The model under review builds one solid part; all positions refer to its coordinate system, in mm. Round coordinates to 2 decimals unless told otherwise and drop trailing zeros. Order: outer loops, then holes, each group sorted by start corner. A loop starts at its lowest first (then second) coordinate and runs counter-clockwise, first axis right, second up. Notation, with made-up numbers: M -13,23 L 15,23 A14 ccw 15,48 Z; hole C 54.5,0 d11. An arc over 180 degrees is marked long. One line per item, written item: value. Start each with the question number.
from build123d import *

# Parameters (mm, degrees)
SKETCH_1_R          = 2
SKETCH_1_R_2        = 1.5
EXTRUDE_1_DEPTH     = 3
SKETCH_2_W          = 80
SKETCH_2_H          = 23
SKETCH_2_H_2        = 10
CUT_EXTRUDE_1_DEPTH = 124.020323524
FILLET_1_R          = 2
FILLET_2_R          = 3
FILLET_3_R          = 1


with BuildPart() as part:
    # 草图1 → 凸台-拉伸1 (new body)
    with BuildSketch(Plane(origin=(0, 0, 0), x_dir=(1, 0, 0), z_dir=(0, 1, 0))):
        Polygon((55, 110), (55, 0), (-55, 0), (-55, 110), (-40, 110), (-40, 55), (40, 55), (40, 110), align=None)
        with Locations(Location((47.5, 32.5, 0), (0, 0, 270))):
            Circle(SKETCH_1_R, mode=Mode.SUBTRACT)
        with Locations(Location((47.5, 7.5, 0), (0, 0, 270))):
            Circle(SKETCH_1_R, mode=Mode.SUBTRACT)
        with Locations(Location((47.5, 79.5, 0), (0, 0, 270))):
            Circle(SKETCH_1_R, mode=Mode.SUBTRACT)
        with Locations(Location((47.5, 102.5, 0), (0, 0, 270))):
            Circle(SKETCH_1_R, mode=Mode.SUBTRACT)
        with Locations(Location((-47.5, 102.5, 0), (0, 0, 90))):
            Circle(SKETCH_1_R, mode=Mode.SUBTRACT)
        with Locations(Location((-47.5, 79.5, 0), (0, 0, 90))):
            Circle(SKETCH_1_R, mode=Mode.SUBTRACT)
        with Locations(Location((-47.5, 7.5, 0), (0, 0, 90))):
            Circle(SKETCH_1_R, mode=Mode.SUBTRACT)
        with Locations(Location((-47.5, 32.5, 0), (0, 0, 90))):
            Circle(SKETCH_1_R, mode=Mode.SUBTRACT)
        with Locations(Location((-32, 36, 0), (0, 0, 270))):
            Circle(SKETCH_1_R_2, mode=Mode.SUBTRACT)
        with Locations(Location((32, 36, 0), (0, 0, 90))):
            Circle(SKETCH_1_R_2, mode=Mode.SUBTRACT)
    extrude(amount=EXTRUDE_1_DEPTH)

    # 草图2 → 切除-拉伸1 (cut, through all)
    with BuildSketch(Plane(origin=(0, 3, 0), x_dir=(1, 0, 0), z_dir=(0, 1, 0))):
        with Locations((0, 21.5)):
            Rectangle(SKETCH_2_W, SKETCH_2_H)
        with Locations((0, 44)):
            Rectangle(SKETCH_2_W, SKETCH_2_H_2)
        with BuildLine():
            Line((-45.5, 70), (-45.5, 42))
            ThreePointArc((-45.5, 42), (-47.5, 40), (-49.5, 42))
            Line((-49.5, 42), (-49.5, 70))
            ThreePointArc((-49.5, 70), (-47.5, 72), (-45.5, 70))
        make_face()
        with BuildLine():
            Line((45.5, 70), (45.5, 42))
            ThreePointArc((45.5, 42), (47.5, 40), (49.5, 42))
            Line((49.5, 42), (49.5, 70))
            ThreePointArc((49.5, 70), (47.5, 72), (45.5, 70))
        make_face()
    extrude(amount=-CUT_EXTRUDE_1_DEPTH, mode=Mode.SUBTRACT)

    # 圆角1
    fillet_1_edges = [part.edges().sort_by_distance(p)[0] for p in [
        (55, 1.5, -110),
        (55, 1.5, 0),
        (-55, 1.5, 0),
        (-55, 1.5, -110),
        (-40, 1.5, -110),
        (-40, 1.5, -55),
        (40, 1.5, -55),
        (40, 1.5, -110),
    ]]
    fillet(fillet_1_edges, radius=FILLET_1_R)

    # 圆角2
    fillet_2_edges = [part.edges().sort_by_distance(p)[0] for p in [
        (-40, 1.5, -33),
        (40, 1.5, -33),
        (40, 1.5, -39),
        (-40, 1.5, -39),
    ]]
    fillet(fillet_2_edges, radius=FILLET_2_R)

    # 圆角3
    fillet_3_edges = [part.edges().sort_by_distance(p)[0] for p in [
        (-40, 1.5, -10),
        (40, 1.5, -10),
        (-40, 1.5, -49),
        (40, 1.5, -49),
    ]]
    fillet(fillet_3_edges, radius=FILLET_3_R)


solid = part.part
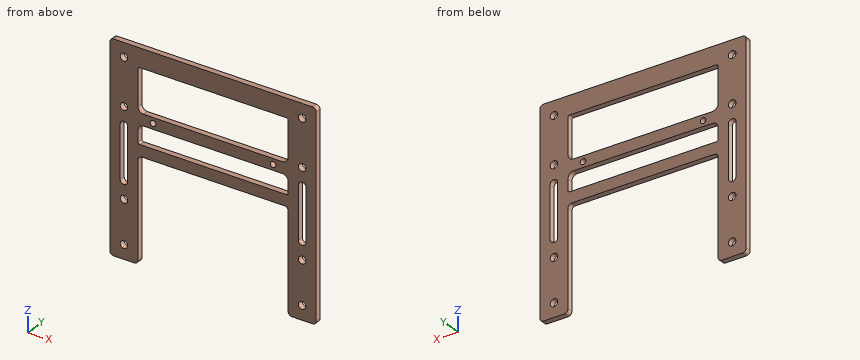
Item 1: Clearance check with a flat-ended pin moving along its axis: P1, Ø1.5, axis at x = 11.5, y = 1, coming from the -Z side. State where the tip first meets the part, or that it passes through.
Item 2: Consider section A-A, the plane x = 32. Give the boundary of the cut face in (y, z).
Item 3: Wall thickness on L1, parallel to X at y = 1.2, z = -36; L2, parallel to Z at x = -47.5, y = 1.6; L3, parallel to Z at x = 21, y = 1.45: over which ranges is each line inside the solid? List them lowest first.
Item 4: Consider section C-C, the plane x = -7. Give the boundary of the cut face in (y, z), then the cut area to 3 significant figures.
Item 5: Consider section D-D, the plane x = 47.5. Give the boundary of the cut face in (y, z).
Item 6: Consider section B-B, the plane z = -45.5. Give the boundary of the cut face in (x, y).
Computed:
1. P1: stops at z = -55
2. outline: M 0,-55 L 3,-55 L 3,-49 L 0,-49 Z; M 0,-39 L 3,-39 L 3,-37.5 L 0,-37.5 Z; M 0,-34.5 L 3,-34.5 L 3,-33 L 0,-33 Z; M 0,-10 L 3,-10 L 3,0 L 0,0 Z
3. L1: x = -55 to -33.5, -30.5 to 30.5, 33.5 to 55
3. L2: z = -110 to -104.5, -100.5 to -81.5, -77.5 to -72, -40 to -34.5, -30.5 to -9.5, -5.5 to 0
3. L3: z = -55 to -49, -39 to -33, -10 to 0
4. outline: M 0,-55 L 3,-55 L 3,-49 L 0,-49 Z; M 0,-39 L 3,-39 L 3,-33 L 0,-33 Z; M 0,-10 L 3,-10 L 3,0 L 0,0 Z
4. area: 66.0 mm^2
5. outline: M 0,-110 L 3,-110 L 3,-104.5 L 0,-104.5 Z; M 0,-100.5 L 3,-100.5 L 3,-81.5 L 0,-81.5 Z; M 0,-77.5 L 3,-77.5 L 3,-72 L 0,-72 Z; M 0,-40 L 3,-40 L 3,-34.5 L 0,-34.5 Z; M 0,-30.5 L 3,-30.5 L 3,-9.5 L 0,-9.5 Z; M 0,-5.5 L 3,-5.5 L 3,0 L 0,0 Z
6. outline: M -55,0 L -49.5,0 L -49.5,3 L -55,3 Z; M -45.5,0 L -40,0 L -40,3 L -45.5,3 Z; M 40,0 L 45.5,0 L 45.5,3 L 40,3 Z; M 49.5,0 L 55,0 L 55,3 L 49.5,3 Z
